from build123d import *
from OCP.BRepFilletAPI import BRepFilletAPI_MakeChamfer

# Parameters (mm, degrees)
SKETCH1_W           = 27.75
SKETCH1_H           = 28
BOSS_EXTRUDE1_DEPTH = 0.84
CUT_EXTRUDE1_REACH  = 21.729
SKETCH2_W           = 6.5
SKETCH2_H           = 9
CHAMFER1_SIZE       = 2
CHAMFER2_SIZE       = 0.36
CHAMFER2_SIZE2      = 3.6
FILLET1_R           = 0.5
FILLET2_R           = 0.25


with BuildPart() as part:
    # Sketch1 → Boss-Extrude1 (new body)
    with BuildSketch(Plane(origin=(0, 0, 0), x_dir=(1, 0, 0), z_dir=(0, 1, 0))):
        Rectangle(SKETCH1_W, SKETCH1_H)
    extrude(amount=BOSS_EXTRUDE1_DEPTH)

    # Sketch2 → Cut-Extrude1 (cut, up to next)
    with BuildSketch(Plane(origin=(0, 0, 0), x_dir=(1, 0, 0), z_dir=(0, 1, 0)), mode=Mode.PRIVATE) as cut_extrude1_sk1:
        with Locations((-10.625, 1.5)):
            Rectangle(SKETCH2_W, SKETCH2_H)
    cut_extrude1_tool1 = extrude(cut_extrude1_sk1.sketch, amount=CUT_EXTRUDE1_REACH, mode=Mode.PRIVATE) & part.part
    # Sketch2 → Cut-Extrude1 (cut, up to next)
    with BuildSketch(Plane(origin=(0, 0, 0), x_dir=(1, 0, 0), z_dir=(0, 1, 0)), mode=Mode.PRIVATE) as cut_extrude1_sk2:
        with Locations((10.625, 1.5)):
            Rectangle(SKETCH2_W, SKETCH2_H)
    cut_extrude1_tool2 = extrude(cut_extrude1_sk2.sketch, amount=CUT_EXTRUDE1_REACH, mode=Mode.PRIVATE) & part.part
    # Sketch2 → Cut-Extrude1 (cut, up to next)
    with BuildSketch(Plane(origin=(0, 0, 0), x_dir=(1, 0, 0), z_dir=(0, 1, 0)), mode=Mode.PRIVATE) as cut_extrude1_sk3:
        Polygon((0, -1.386751346), (2.5, 2.943375673), (-2.5, 2.943375673), align=None)
    cut_extrude1_tool3 = extrude(cut_extrude1_sk3.sketch, amount=CUT_EXTRUDE1_REACH, mode=Mode.PRIVATE) & part.part
    add(cut_extrude1_tool1.solids().sort_by_distance((-10.625, 0, -1.5))[0], mode=Mode.SUBTRACT)
    add(cut_extrude1_tool2.solids().sort_by_distance((10.625, 0, -1.5))[0], mode=Mode.SUBTRACT)
    add(cut_extrude1_tool3.solids().sort_by_distance((0, 0, -1.5))[0], mode=Mode.SUBTRACT)

    # Chamfer1
    chamfer1_edges = [part.edges().sort_by_distance(p)[0] for p in [
        (-13.875, 0.42, -14),
        (13.875, 0.42, -14),
        (13.875, 0.42, 14),
        (-13.875, 0.42, 14),
    ]]
    chamfer(chamfer1_edges, length=CHAMFER1_SIZE)

    # Chamfer2: one chamfer whose edges measure the first distance from different faces: ONE call of the kernel's chamfer builder (chamfer() names one face for all edges)
    chamfer2_edges_1 = [part.edges().sort_by_distance(p)[0] for p in [
        (0, 0.84, -14),
    ]]
    chamfer2_side_1 = [part.faces().sort_by_distance(p)[0] for p in [
        (0, 0.42, -14),
    ]]
    chamfer2_edges_2 = [part.edges().sort_by_distance(p)[0] for p in [
        (0, 0.84, 14),
    ]]
    chamfer2_side_2 = [part.faces().sort_by_distance(p)[0] for p in [
        (0, 0.42, 14),
    ]]
    chamfer2 = BRepFilletAPI_MakeChamfer(part.part.solid().wrapped)
    for e in chamfer2_edges_1:
        chamfer2.Add(CHAMFER2_SIZE, CHAMFER2_SIZE2, e.wrapped, chamfer2_side_1[0].wrapped)  # the first distance lies on this face
    for e in chamfer2_edges_2:
        chamfer2.Add(CHAMFER2_SIZE, CHAMFER2_SIZE2, e.wrapped, chamfer2_side_2[0].wrapped)  # the first distance lies on this face
    add(Compound.cast(chamfer2.Shape()), mode=Mode.REPLACE)

    # Fillet1
    fillet1_edges = [part.edges().sort_by_distance(p)[0] for p in [
        (-7.375, 0.42, 3),
        (-7.375, 0.42, -6),
        (-13.875, 0.42, -6),
        (-13.875, 0.42, 3),
        (13.875, 0.42, 3),
        (13.875, 0.42, -6),
        (7.375, 0.42, -6),
        (7.375, 0.42, 3),
        (11.875, 0.24, 14),
        (-13.875, 0.34, 12),
        (-11.875, 0.24, -14),
        (13.875, 0.34, -12),
        (-13.875, 0.34, -12),
        (11.875, 0.24, -14),
        (13.875, 0.34, 12),
        (-11.875, 0.24, 14),
    ]]
    fillet(fillet1_edges, radius=FILLET1_R)

    # Fillet2
    fillet2_edges = [part.edges().sort_by_distance(p)[0] for p in [
        (-2.5, 0.42, -2.943375673),
        (0, 0.42, 1.386751346),
        (2.5, 0.42, -2.943375673),
    ]]
    fillet(fillet2_edges, radius=FILLET2_R)


solid = part.part
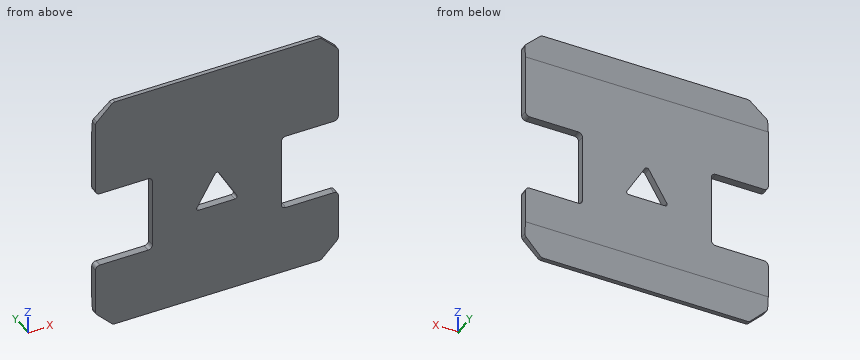
Design review of the part built by this model. Coordinates are the model's own, in mm. Round coordinates to 2 decimals unless told otherwise and drop trailing zeros. Write each loop counter-clockwise with the first axis right and the second up, starting at its lowest first coordinate (ties: lowest second). Pieces come first, ordered by that corner, then holes.
Item 1: Consider section D-D on z = -3.75. Give the boundary of the cut face in (x, y) (3 decimals).
Item 2: Consider section A-A on x = 9.25. Give the boundary of the cut face in (y, z).
Item 3: Consider section C-C on x = 4.5. Give the boundary of the cut face in (y, z), and give its area (3 significant figures).
Item 4: Wall thickness on L1, parallel to Z at x = -10, y = 0.4; L2, parallel to X at y = 0.5, z = -4 (3 decimals); L3, parallel to X at y = 0.6, z = -0.5 (3 decimals): over which ranges is each line inside the solid? List them lowest first.
Item 5: Consider section B-B on z = 0. Give the boundary of the cut face in (x, y) (3 decimals).
Check values:
1. outline: (-7.375, 0) - (7.375, 0) - (7.375, 0.84) - (-7.375, 0.84) - close
2. outline: (0, -14) - (0.48, -14) - (0.84, -10.4) - (0.84, -6) - (0, -6) - close; (0, 3) - (0.84, 3) - (0.84, 10.4) - (0.48, 14) - (0, 14) - close
3. outline: (0, -14) - (0.48, -14) - (0.84, -10.4) - (0.84, 10.4) - (0.48, 14) - (0, 14) - close
3. area: 22.2 mm2
4. L1: z = -14 to -6, 3 to 14
4. L2: x = -7.375 to 7.375
4. L3: x = -7.375 to -1.089, 1.089 to 7.375
5. outline: (-7.375, 0) - (-0.801, 0) - (-0.801, 0.84) - (-7.375, 0.84) - close; (0.801, 0) - (7.375, 0) - (7.375, 0.84) - (0.801, 0.84) - close
